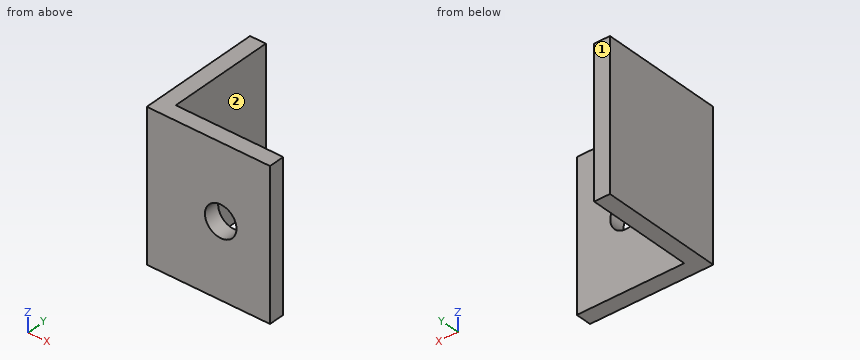
```python
from build123d import *

# Parameters (mm, degrees)
BOSS_EXTRUDE1_DEPTH = 15
SKETCH2_R           = 1.6
CUT_EXTRUDE1_DEPTH  = 23.362021376


with BuildPart() as part:
    # Sketch1 → Boss-Extrude1 (new body)
    with BuildSketch(Plane.XY):
        Polygon((0, 0), (0, 12.5), (1.6, 12.5), (1.6, 1.6), (12.5, 1.6), (12.5, 0), align=None)
    extrude(amount=BOSS_EXTRUDE1_DEPTH)

    # Sketch2 → Cut-Extrude1 (cut, through all)
    with BuildSketch(Plane(origin=(0, 1.6, 0), x_dir=(1, 0, 0), z_dir=(0, 1, 0))):
        with Locations(Location((7.5, -7.5, 0), (0, 0, 180))):
            Circle(SKETCH2_R)
    extrude(amount=-CUT_EXTRUDE1_DEPTH, mode=Mode.SUBTRACT)


solid = part.part
```
For this review, take the finished solid that the model builds, in its own axes (mm). Face numbers are marked on the shaded views. A direction names the side the tool comes from. Round coordinates to 2 decimals unless told otherwise and drop trailing zeros. Write each loop counter-clockwise with the first axis right and the second up, starting at its lowest first coordinate (ties: lowest second). Pieces come first, ordered by that corner, then holes. Notation, with made-up numbers: (-31, 55) -> (-7, 55) arc R26 ccw to (-7, 75) -> close; hole circle Ø10 at (69.25, -17). An arc over 180 degrees is marked (long way). One line per question, with ' | ' between items. Start each with the question number.
1) For pin 1 Ø4 at (x, z) = (7.5, 7.5) entering from +Y; pin 2 Ø2 at (x, z) = (7.5, 6) entering from -Y; pin 3 Ø1.5 at (y, z) = (6, 12.5) entering from +X, all flat-tipped, find the tip position at first contact; note any pin that passes through.
2) Add section A-A (x = 7.5). Write out the cut boundary in (y, z), and give its area (3 significant figures).
3) Add section C-C (z = 10.5). Write out the cut boundary in (x, y).
4) Wall thickness on line 1 along Z through (x, y) = (7.5, 0.7); line 2 along X through (y, z) = (6.75, 1.5): over which ranges is each line inside the solid? List them lowest first.
5) Machinability: for the marked faces 1 and 2, which of the approach directions +Z, -Z, +X, -X, +Y, -Y give a long, thin tool a straight path to every point of the face, cutting with its end or side? Answer none if there is none.
6) Add section B-B (z = 8.25). Write out the cut boundary in (x, y), and give its area (3 significant figures).
7) Add section D-D (y = 5). Write out the cut boundary in (x, z).
Reported:
1) pin 1: stops at y = 1.6 | pin 2: stops at y = 0 | pin 3: stops at x = 1.6
2) outline: (0, 0) -> (1.6, 0) -> (1.6, 5.9) -> (0, 5.9) -> close; (0, 9.1) -> (1.6, 9.1) -> (1.6, 15) -> (0, 15) -> close | area: 18.9 mm²
3) outline: (0, 0) -> (12.5, 0) -> (12.5, 1.6) -> (1.6, 1.6) -> (1.6, 12.5) -> (0, 12.5) -> close
4) line 1: z = 0 to 5.9, 9.1 to 15 | line 2: x = 0 to 1.6
5) face 1: +Z, -Z, +X, -X, +Y | face 2: +Z, -Z, +X, +Y
6) outline: (0, 0) -> (6.09, 0) -> (6.09, 1.6) -> (1.6, 1.6) -> (1.6, 12.5) -> (0, 12.5) -> close; (8.91, 0) -> (12.5, 0) -> (12.5, 1.6) -> (8.91, 1.6) -> close | area: 32.9 mm²
7) outline: (0, 0) -> (1.6, 0) -> (1.6, 15) -> (0, 15) -> close
